Part print with two shaded views. Sizes in mm from the minimum x, y, z corner. A direction names the side the tool comes from. Round coordinates to 2 decimals unless told otherwise and drop trailing zeros. Write each loop counter-clockwise with the first axis right and the second up, starting at its lowest first coordinate (ties: lowest second). Pieces come first, ordered by that corner, then holes. Notation, with made-up numbers: (-32.75, 31.5) -> (-19.75, 31.5) arc R30 cw to (-19.75, 58.5) -> close; hole circle Ø8 at (-36, 27.5). An arc over 180 degrees is marked (long way). Return JSON: item names as keys, results as strings. Group by question number.
(1) Drill centre lines: L1, parallel to Z at x = 27, y = 8.5; L2, parallel to X at y = 33.5, z = 7; L3, parallel to X at y = 38, z = 11 (1 decimal). Where is each one in solid material? Low to high. Write a range as from..to.
(2) Saw through at A-A (z = 11.5). List the corners of the cut face in (x, y) (1 decimal), plus the area to 3 significant figures.
(3) Tool access for the marked faces 4 and 5: list every direction of +Z, -Z, +X, -X, +Y, -Y with a clear straight run to the whole face (end or side of a thin tool).
(4) Drop flat-ended pins along their axis: pin 1 Ø2 at (y, z) = (54, 2) entering from -X; pin 2 Ø4 at (y, z) = (60, 3) entering from -X; pin 3 Ø1 at (x, z) = (43, 5) entering from -Y (1 decimal). Give the stop position or say it passes through.
(5) Saw through at B-B (x = 10.5). List the corners of the cut face in (y, z).
(6) Mould opens along Y. For the marked faces 1, 2 and 3 say: +Y half, -Y half, draft (parallel to the pull), parting line (faces both ways), or undercut.
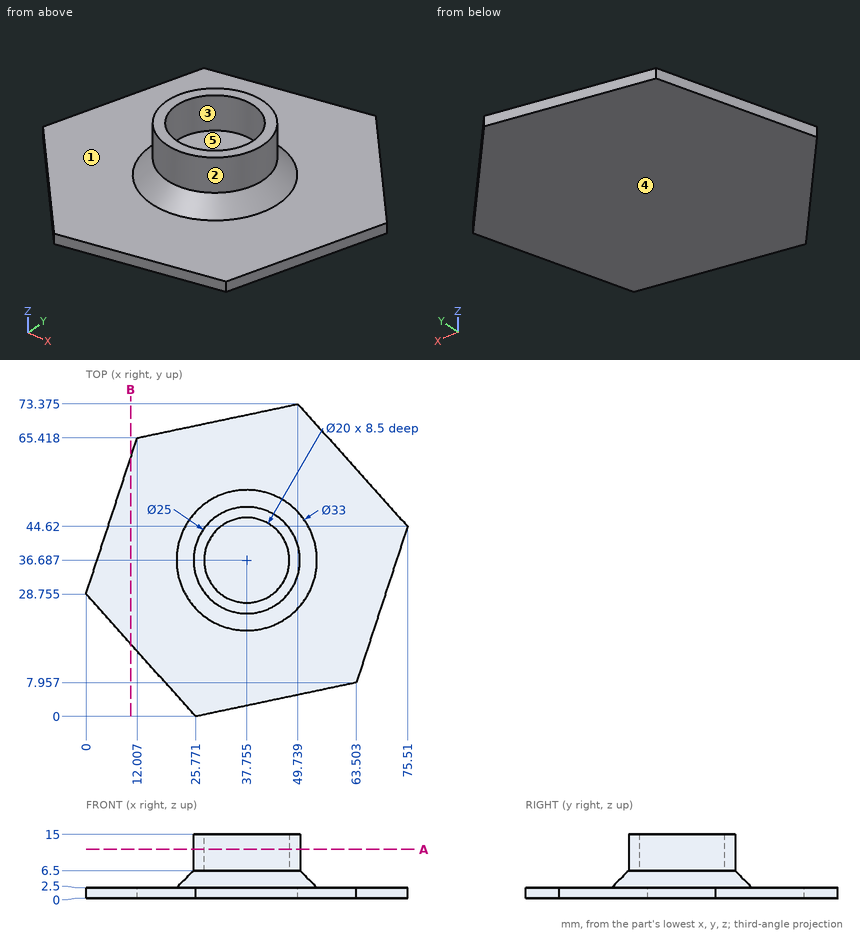
Computed values:
{
 "1": {"L1": "0..2.5", "L2": "25.67..28.28, 47.23..49.84", "L3": "25.3..27.8, 47.7..50.2"},
 "2": {"outline": "circle Ø25 at (37.8, 36.7); hole circle Ø20 at (37.8, 36.7)", "area": "177 mm2"},
 "3": {"face 4": "-Z, +X, -X, +Y, -Y", "face 5": "+Z"},
 "4": {"pin 1": "x = 7.94", "pin 2": "x = 9.6", "pin 3": "y = 23.1"},
 "5": {"outline": "(17.04, 0) -> (60.82, 0) -> (60.82, 2.5) -> (17.04, 2.5) -> close"},
 "6": {"face 1": "draft", "face 2": "parting line", "face 3": "undercut"}
}
